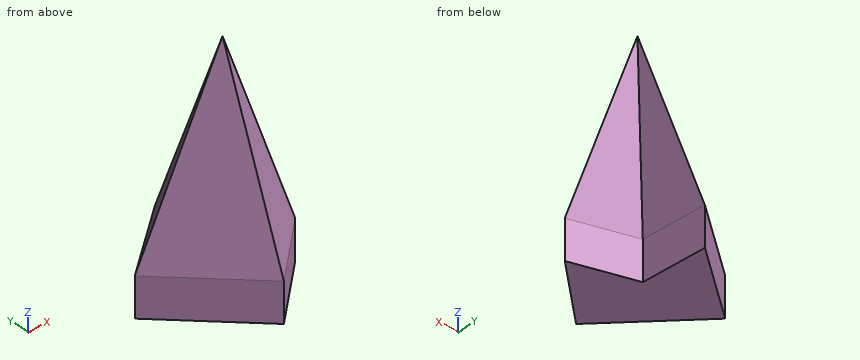
```python
from build123d import *

# Parameters (mm, degrees)
F1_DEPTH = 25


with BuildPart() as f1:
    # F0 (on Top) → F1 (new body)
    with BuildSketch(Plane.XY):
        Polygon((3.729509, 7.889344), (0, 47.192626), (-43.893445, 12.479508), (5.163935, -37.151642), (41.885249, -4.159836), align=None)
    extrude(amount=F1_DEPTH)

    # F1_face (on face) → F4 section 0
    with BuildSketch(Plane(origin=(-3.684593, 1.905517, 25), x_dir=(1, 0, 0), z_dir=(0, 0, 1)), mode=Mode.PRIVATE) as f4_s0:
        Polygon((45.569842, -6.065353), (7.414102, 5.983827), (3.684593, 45.287109), (-40.208852, 10.573991), (8.848528, -39.057159), align=None)
    loft([f4_s0.sketch, Vertex(0, 0, 150)])


solid = f1.part
```
The model under review builds one solid part; all positions refer to its coordinate system, in mm. Coordinates: 2 decimals unless noted, no trailing zeros. Write each loop counter-clockwise with the first axis right and the second up, starting at its lowest first coordinate (ties: lowest second). Pieces come first, ordered by that corner, then holes. Notation, with made-up numbers: (-31, 39) -> (28, 39) arc R34 cw to (28, 76) -> close; hole circle Ø3 at (72, 7.5). An arc over 180 degrees is marked (long way). One line per item, written item: value. Start each with the question number.
Q1. Add section A-A, the plane z = 10. Give the boundary of the cut face in (x, y), then the cut area to 3 significant figures.
Q2. Clearance check with flat-ended pins moving along their axes: P1, Ø12, axis at y = -18.5, z = 81, coming from the +X side; P2, Ø10, axis at y = -13, z = 36, coming from the -X side; P3, Ø8, axis at y = -22, z = 82.5, coming from the +X side. State where each tip first meets the part, or that it passes through.
Q3. Add section B-B, the plane x = -26. Give the boundary of the cut face in (y, z), then the cut area to 3 significant figures.
Q4. To check wall thickness, follow probe 1 along Y at (x, z) = (13.5, 57.5); probe 2 along Y at (x, z) = (11.5, 26.5); probe 3 along X at (y, z) = (-10.5, 97.5). State the ranges of each line that lie inside material, in increasing order.
Response:
1. outline: (-43.89, 12.48) -> (5.16, -37.15) -> (41.89, -4.16) -> (3.73, 7.89) -> (0, 47.19) -> close
1. area: 2,850 mm²
2. P1: x = 12.13
2. P2: x = -21.03
2. P3: x = 5.33
3. outline: (-5.62, 0) -> (26.63, 0) -> (26.63, 25) -> (7.39, 75.96) -> (-5.62, 25) -> close
3. area: 1,630 mm²
4. probe 1: -18.8 to 2.45
4. probe 2: -30.96 to 5.33
4. probe 3: -2.88 to 7.85
